Here's how the part is built. I have some questions about the finished solid (model axes, mm). A direction names the side the tool comes from. Give positions to 0.01 mm unless a question says otherwise; leave off trailing zeros. Write each loop counter-clockwise with the first axis right and the second up, starting at its lowest first coordinate (ties: lowest second). Pieces come first, ordered by that corner, then holes. Notation, with made-up numbers: (46.25, -32.75) - (63.25, -32.75) arc R21 cw to (63.25, -19.75) - close; hole circle Ø4 at (41, 81.5). An arc over 180 degrees is marked (long way). One line per item, written item: value. Start each with the question number.
1) I'm going to push flat-ended pins straight in: P1, Ø1.6, axis at y = 153.5, z = 43.5, coming from the +X side; P2, Ø5, axis at x = 48, y = 35, coming from the +Z side. Where does each tip first touch, or does it pass through?
2) Imagine slicing it at D-D on x = 109. Write out the boundary of the cut face in (y, z).
3) On a 3-axis mill with a long thin cutter (end or side, diameter ignored), from which of +Z, -Z, +X, -X, +Y, -Y can I reach the whole of each face in a straight line? I mean faces 1 (the flat face through (1, 152.4, 234)), 2 (the flat face through (1, 152.4, -233)), 3 (the flat face through (-142, 152.4, 3)). Say none if no direction works.
4) Imagine slicing it at A-A on x = 48. Write out the boundary of the cut face in (y, z) (1 decimal), plus the area to 3 significant figures.
5) Imagine slicing it at B-B on x = 1. Write out the boundary of the cut face in (y, z) (1 decimal).
6) Please list where these lines run through material, in increasing order: L1, parallel to Z at x = 27.5, y = -107.5; L2, parallel to Y at x = -131.5, z = -158.5; L3, parallel to Y at x = -68, z = -211 (3 decimals). Write a range as [from, to].
7) Imagine slicing it at C-C on y = -123. Write out the boundary of the cut face in (x, z) (1 decimal), plus the area to 3 significant figures.
from build123d import *

# Parameters (mm, degrees)
F0_W     = 412.75
F0_H     = 304.8
F1_DEPTH = 204.7875
F3_DEPTH = 3.175


with BuildPart() as f1:
    # F0 (on Top) → F1 (new body, symmetric)
    with BuildSketch(Plane.XY):
        Rectangle(F0_W, F0_H)
    extrude(amount=F1_DEPTH, both=True)

    # F2 (on face) → F3 (join)
    with BuildSketch(Plane(origin=(0, 152.4, 0), x_dir=(-1, 0, 0), z_dir=(0, 1, 0))):
        with BuildLine():
            ThreePointArc((76.2, 249.2375), (72.4802561211, 258.2177561211), (63.5, 261.9375))
            Line((63.5, 261.9375), (-63.5, 261.9375))
            ThreePointArc((-63.5, 261.9375), (-72.4802561211, 258.2177561211), (-76.2, 249.2375))
            Line((-76.2, 249.2375), (-76.2, -249.2375))
            ThreePointArc((-76.2, -249.2375), (-72.4802561211, -258.2177561211), (-63.5, -261.9375))
            Line((-63.5, -261.9375), (63.5, -261.9375))
            ThreePointArc((63.5, -261.9375), (72.4802561211, -258.2177561211), (76.2, -249.2375))
            Line((76.2, -249.2375), (76.2, 249.2375))
        make_face()
        with BuildLine():
            Line((-64.29375, -227.80625), (-24.60625, -227.80625))
            ThreePointArc((-24.60625, -227.80625), (-19.05, -233.3625), (-24.60625, -238.91875))
            Line((-24.60625, -238.91875), (-64.29375, -238.91875))
            ThreePointArc((-64.29375, -238.91875), (-69.85, -233.3625), (-64.29375, -227.80625))
        make_face(mode=Mode.SUBTRACT)
        with BuildLine():
            Line((24.60625, -227.80625), (64.29375, -227.80625))
            ThreePointArc((64.29375, -227.80625), (69.85, -233.3625), (64.29375, -238.91875))
            Line((64.29375, -238.91875), (24.60625, -238.91875))
            ThreePointArc((24.60625, -238.91875), (19.05, -233.3625), (24.60625, -227.80625))
        make_face(mode=Mode.SUBTRACT)
        with BuildLine():
            Line((-64.29375, 238.91875), (-24.60625, 238.91875))
            ThreePointArc((-24.60625, 238.91875), (-19.05, 233.3625), (-24.60625, 227.80625))
            Line((-24.60625, 227.80625), (-64.29375, 227.80625))
            ThreePointArc((-64.29375, 227.80625), (-69.85, 233.3625), (-64.29375, 238.91875))
        make_face(mode=Mode.SUBTRACT)
        with BuildLine():
            Line((24.60625, 238.91875), (64.29375, 238.91875))
            ThreePointArc((64.29375, 238.91875), (69.85, 233.3625), (64.29375, 227.80625))
            Line((64.29375, 227.80625), (24.60625, 227.80625))
            ThreePointArc((24.60625, 227.80625), (19.05, 233.3625), (24.60625, 238.91875))
        make_face(mode=Mode.SUBTRACT)
    extrude(amount=F3_DEPTH)


solid = f1.part
Numbers:
1. P1: x = 76.2
1. P2: z = 204.79
2. outline: (-152.4, -204.79) - (152.4, -204.79) - (152.4, 204.79) - (-152.4, 204.79) - close
3. face 1: +Z, +X, -X, -Y
3. face 2: -Z, +X, -X, -Y
3. face 3: +Z, -Z, -X, +Y
4. outline: (-152.4, -204.8) - (152.4, -204.8) - (152.4, -227.8) - (155.6, -227.8) - (155.6, 227.8) - (152.4, 227.8) - (152.4, 204.8) - (-152.4, 204.8) - close; (152.4, -261.9) - (155.6, -261.9) - (155.6, -238.9) - (152.4, -238.9) - close; (152.4, 238.9) - (155.6, 238.9) - (155.6, 261.9) - (152.4, 261.9) - close
4. area: 126,000 mm^2
5. outline: (-152.4, -204.8) - (152.4, -204.8) - (152.4, -261.9) - (155.6, -261.9) - (155.6, 261.9) - (152.4, 261.9) - (152.4, 204.8) - (-152.4, 204.8) - close
6. L1: [-204.79, 204.79]
6. L2: [-152.4, 152.4]
6. L3: [152.4, 155.575]
7. outline: (-206.4, -204.8) - (206.4, -204.8) - (206.4, 204.8) - (-206.4, 204.8) - close
7. area: 169,000 mm^2
